Geometry check sheet. Reference: the model listing, model coordinates, mm. Face numbers are marked on the shaded views. A direction names the side the tool comes from. Round coordinates to 2 decimals unless told otherwise and drop trailing zeros. Write each loop counter-clockwise with the first axis right and the second up, starting at its lowest first coordinate (ties: lowest second). Pieces come first, ordered by that corner, then holes. Notation, with made-up numbers: M -12,24 L 23,24 A15 ccw 23,39 Z; hole C 58,-31.5 d5. An arc over 180 degrees is marked long. Use a Markdown table: item, result.
Solid Edge part; units mm, degrees
sketch "Sketch1" plane through (0, 0, 0) normal (0, 0, 1) x (1, 0, 0)
  line L0 (0, 15) -> (15, 15)
  line L1 (15, 15) -> (15, -15)
  line L2 (15, -15) -> (-15, -15)
  line L3 (-15, -15) -> (-15, 15)
  line L4 (-15, 15) -> (0, 15)
extrude "Protrusion1" add sketch "Sketch1" along normal blind 2
sketch "Sketch2" plane through (0, 0, 2) normal (0, 0, 1) x (1, 0, 0)
  line L0 (10, 0) -> (10, 10)
  line L1 (10, 10) -> (-10, 10)
  line L2 (-10, 10) -> (-10, -10)
  line L3 (-10, -10) -> (10, -10)
  line L4 (10, -10) -> (10, 0)
extrude "ExtrudedProtrusion_2" add sketch "Sketch2" along normal blind 12
sketch "Sketch3" plane through (0, 0, 2) normal (0, 0, 1) x (1, 0, 0)
  circle A0 centre (-12.5, -12.5) radius 1.5
  circle A1 centre (12.5, -12.5) radius 1.5
  circle A2 centre (12.5, 12.5) radius 1.5
  circle A3 centre (-12.5, 12.5) radius 1.5
extrude "ExtrudedCutout_1" cut sketch "Sketch3" against normal blind 2
sketch "Sketch4" plane through (0, 0, 14) normal (0, 0, 1) x (1, 0, 0)
  circle A0 centre (0, 0) radius 2.6
extrude "ExtrudedCutout_2" cut sketch "Sketch4" against normal blind 10
fillet "Round_1" radius 5 8 edges at (-10, -10, 8) (-10, 10, 8) (10, -10, 8) (10, 10, 8) (0, 10, 14) (10, 0, 14) (0, -10, 14) (-10, 0, 14)
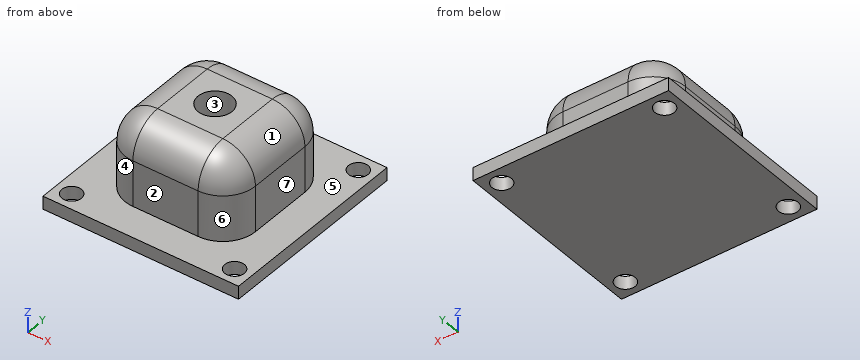
Item 1: Cross-section at D-D, the plane y = -1. Record the cut outline in (x, z), and give its area (3 significant figures).
Outcome:
| item | result |
|---|---|
| outline | M -15,0 L 15,0 L 15,2 L 10,2 L 10,9 A5 ccw 5,14 L 2.4,14 L 2.4,4 L -2.4,4 L -2.4,14 L -5,14 A5 ccw -10,9 L -10,2 L -15,2 Z |
| area | 241 mm2 |
Item 2: Material ranges on line 1 along Y through (x, z) = (12.5, 0.85); line 2 along X through (y, z) = (5.25, 2.25); line 3 along Y through (x, z) = (3, 4.5), recorded low to high. Write a range as from..to.
Outcome:
| item | result |
|---|---|
| line 1 | y = -15..-14, -11..11, 14..15 |
| line 2 | x = -9.99..9.99 |
| line 3 | y = -10..10 |
Item 3: Mould release check, pull along X, two halves, no side actions. Record for the marked faces 1, 2, 3 and 4: +X half, -X half, draft (parallel to the pull), parting line (faces both ways), or undercut.
Outcome:
| item | result |
|---|---|
| face 1 | +X half |
| face 2 | draft |
| face 3 | undercut |
| face 4 | -X half |
Item 4: Cross-section at A-A, the plane y = -12.5. Record the cut outline in (x, z), and give its area (3 significant figures).
Outcome:
| item | result |
|---|---|
| outline | M -15,0 L -14,0 L -14,2 L -15,2 Z; M -11,0 L 11,0 L 11,2 L -11,2 Z; M 14,0 L 15,0 L 15,2 L 14,2 Z |
| area | 48.0 mm2 |
Item 5: Go/stop test with flat-tipped pins: pin 1 (2 mm diameter, centred on x = -8, z = 10.5, fed in from -Y); pin 2 (3.5 mm diameter, centred on x = 1, z = 4.5, fed in from -Y); pin 3 (1.5 mm diameter, centred on x = -4, y = 7.5, fed in from +Z). Record where each tip stops, or that it passes through.
Outcome:
| item | result |
|---|---|
| pin 1 | stops at y = -9.41 |
| pin 2 | stops at y = -10 |
| pin 3 | stops at z = 13.68 |
Item 6: Access from +Z, -Z, +X, -X, +Y, -Y to the whole of each face (thin tool, end or side, straight path). Record for the marked faces 5, 6 and 7.
Outcome:
| item | result |
|---|---|
| face 5 | +Z |
| face 6 | +Z, +X, -Y |
| face 7 | +Z, +X, +Y, -Y |
Item 7: Cross-section at C-C, the plane z = 2.5. Record the cut outline in (x, y).
Outcome:
| item | result |
|---|---|
| outline | M -10,-5 A5 ccw -5,-10 L 5,-10 A5 ccw 10,-5 L 10,5 A5 ccw 5,10 L -5,10 A5 ccw -10,5 Z |
